Autodesk Inventor part; units mm, degrees
ref_plane "YZ Plane" through (0, 0, 0) normal (1, 0, 0) x (0, 1, 0)
ref_plane "XZ Plane" through (0, 0, 0) normal (0, 1, 0) x (-1, 0, 0)
ref_plane "XY Plane" through (0, 0, 0) normal (0, 0, 1) x (1, 0, 0)
sketch "Sketch1" plane through (0, 0, 0) normal (1, 0, 0) x (0, 1, 0)
  line L0 (0, 0) -> (6.5, 0)
  line L1 (6.5, 0) -> (6.5, -13.5)
  line L2 (6.5, -13.5) -> (0, -13.5)
  line L3 (0, -13.5) -> (0, 0)
  dimension "d0" = 6.5
  dimension "d1" = 13.5
extrude "Extrusion1" add sketch "Sketch1" along normal blind 6.1
sketch "Sketch2" plane through (0, 0, 0) normal (-1, 0, 0) x (0, 0, 1)
  line L0 (-13.5, 3.5) -> (0, 3.5)
  line L1 (0, 3.5) -> (0, 6.5)
  line L2 (0, 6.5) -> (-13.5, 6.5)
  line L3 (-13.5, 6.5) -> (-13.5, 3.5)
  line L4 (0, 6.5) -> (0, 0)
  line L5 (-13.5, 6.5) -> (0, 6.5)
  dimension "d4" = 3
  dimension "d5" = 13.5
  dimension "d6" = 0
  dimension "d7" = 0
extrude "Extrusion2" add sketch "Sketch2" along normal blind 14.5
sketch "Sketch3" plane through (6.1, 6.5, 0) normal (0, 1, 0) x (1, 0, 0)
  circle A0 centre (-14.85, 6.75) radius 2.25
  line L0 (-20.6, 0) -> (-20.6, 13.5)
  line L1 (-20.6, 0) -> (0, 0)
  point P0 (-6.1, 0)
  dimension "d10" = 4.5
  dimension "d11" = 5.75
  dimension "d12" = 6.75
extrude "Extrusion3" cut sketch "Sketch3" against normal blind 14.5
sketch "Sketch4" plane through (6.1, 0, -13.5) normal (0, 0, -1) x (-1, 0, 0)
  point P0 (6.1, 0)
properties part number "gear support attachment"
Verification items for the finished model (mm, model axes). A direction names the side the tool comes from. Coordinates: 2 decimals unless noted, no trailing zeros. Order: outer loops, then holes, each group sorted by start corner. A loop starts at its lowest first (then second) coordinate and runs counter-clockwise, first axis right, second up.
1. Release check for a two-part mould opening along Z. For faces 3 (the face through (-2, 4, -13.5)), 4 (the face through (-10.41, 5.02, -8.27)), 5 (the face through (-4, 6.5, -7)) record: +Z half, -Z half, draft (parallel to the pull), parting line (faces both ways), or undercut.
Results found:
face 3: -Z half
face 4: undercut
face 5: draft
2. Sectioned sample at B-B, the plane x = -8.75. Record the cut outline in (y, z), and give its area (3 significant figures).
Results found:
outline: (3.5, -13.5) - (6.5, -13.5) - (6.5, -9) - (3.5, -9) - close; (3.5, -4.5) - (6.5, -4.5) - (6.5, 0) - (3.5, 0) - close
area: 27.0 mm2
3. Sectioned sample at A-A, the plane z = -6.75. Record the cut outline in (x, y).
Results found:
outline: (-14.5, 3.5) - (-11, 3.5) - (-11, 6.5) - (-14.5, 6.5) - close; (-6.5, 3.5) - (0, 3.5) - (0, 0) - (6.1, 0) - (6.1, 6.5) - (-6.5, 6.5) - close
4. Sectioned sample at D-D, the plane z = -2.5. Record the cut outline in (x, y).
Results found:
outline: (-14.5, 3.5) - (0, 3.5) - (0, 0) - (6.1, 0) - (6.1, 6.5) - (-14.5, 6.5) - close
5. Set-up check for faces 1 (the face through (-2, 4, 0)), 2 (the face through (0, 2, -7)): record each of +Z, -Z, +X, -X, +Y, -Y from which the full face is reachable in a straight line by a thin tool's end or side.
Results found:
face 1: +Z, +X, -X, +Y, -Y
face 2: +Z, -Z, -X, -Y
6. Go/stop test with a flat-tipped pin: pin 1 Ø4 at (x, z) = (-2.5, -8.5) entering from -Y. Record where the tip stops, or that it passes through.
Results found:
pin 1: stops at y = 3.5
7. Scan lines: line 1 (X direction, y = 4.1, z = -6.75); line 2 (Y direction, x = -13.5, z = -9.75); line 3 (Z direction, x = -8.75, y = 5.15). Record each from-to range of solid material in increasing order.
Results found:
line 1: x = -14.5 to -11, -6.5 to 6.1
line 2: y = 3.5 to 6.5
line 3: z = -13.5 to -9, -4.5 to 0
8. Sectioned sample at C-C, the plane y = 4.75. Record the cut outline in (x, z).
Results found:
outline: (-14.5, -13.5) - (6.1, -13.5) - (6.1, 0) - (-14.5, 0) - close; hole circle Ø4.5 at (-8.75, -6.75)
